Build history of the part. All positions in model axes, mm. A direction names the side the tool comes from. Give positions to 0.01 mm unless a question says otherwise; leave off trailing zeros. Order: outer loops, then holes, each group sorted by start corner. A loop starts at its lowest first (then second) coordinate and runs counter-clockwise, first axis right, second up. Notation, with made-up numbers: M -10,78 L 43,78 A35 ccw 43,110 Z; hole C -36.5,88 d8. An arc over 180 degrees is marked long. One line per item, written item: value.
from build123d import *

# Parameters (mm, degrees)
F0_W     = 42
F0_H     = 42
F1_DEPTH = 5
F3_D     = 5
F4_W     = 42
F4_H     = 5
F5_DEPTH = 5
F6_W     = 42
F6_H     = 5
F7_DEPTH = 20
F8_W     = 42
F8_H     = 5
F8_H_2   = 25
F9_DEPTH = 5
F11_D    = 5
F13_D    = 25


with BuildPart() as f1:
    # F0 (on Top) → F1 (new body)
    with BuildSketch(Plane.XY):
        Rectangle(F0_W, F0_H)
    extrude(amount=F1_DEPTH)

    # F3 (through all)
    with Locations(Plane.XY.offset(5)):
        with Locations((-15.5, 15.5), (15.5, 15.5), (15.5, -15.5), (-15.5, -15.5)):
            Hole(F3_D / 2)

    # F4 (on face) → F5 (join)
    with BuildSketch(Plane(origin=(0, 21, 0), x_dir=(-1, 0, 0), z_dir=(0, 1, 0))):
        with Locations((0, 2.5)):
            Rectangle(F4_W, F4_H)
    extrude(amount=F5_DEPTH)

    # F6 (on face) → F7 (join)
    with BuildSketch(Plane(origin=(0, 0, 0), x_dir=(1, 0, 0), z_dir=(0, 0, -1))):
        with Locations((0, -23.5)):
            Rectangle(F6_W, F6_H)
    extrude(amount=F7_DEPTH)

    # F8 (on face) → F9 (join)
    with BuildSketch(Plane(origin=(0, 0, -20), x_dir=(1, 0, 0), z_dir=(0, 0, -1))):
        with Locations((0, -23.5)):
            Rectangle(F8_W, F8_H)
        with Locations((0, -38.5)):
            Rectangle(F8_W, F8_H_2)
    extrude(amount=F9_DEPTH)

    # F11 (through all)
    with Locations(Plane(origin=(0, 0, -25), x_dir=(1, 0, 0), z_dir=(0, 0, -1))):
        with Locations((-16.56834, -31.176092), (16.56834, -31.176092), (16.56834, -45.494268), (-16.56834, -45.494268)):
            Hole(F11_D / 2)

    # F13 (through all)
    with Locations(Plane(origin=(0, 0, 0), x_dir=(1, 0, 0), z_dir=(0, 0, -1))):
        with Locations((0, 0)):
            Hole(F13_D / 2)


solid = f1.part
1) Saw through at C-C, the plane y = 0. Write the cut outline in (x, z), then the cut area to 3 significant figures.
Check values:
outline: M -21,0 L -12.5,0 L -12.5,5 L -21,5 Z; M 12.5,0 L 21,0 L 21,5 L 12.5,5 Z
area: 85.0 mm^2
2) Saw through at B-B, the plane y = -15.5. Write the cut outline in (x, z).
Check values:
outline: M -21,0 L -18,0 L -18,5 L -21,5 Z; M -13,0 L 13,0 L 13,5 L -13,5 Z; M 18,0 L 21,0 L 21,5 L 18,5 Z
3) Tool access for faces 4 (the face through (0, 26, -7)), 5 (the face through (-9, 9, 0)), 6 (the face through (-17.912, 43.386, -22.465)): list every direction of +Z, -Z, +X, -X, +Y, -Y with a clear straight run to the whole face (end or side of a thin tool).
Check values:
face 4: +Z, +X, -X, +Y
face 5: -Z, +X, -X, -Y
face 6: +Z, -Z
4) Saw through at A-A, the plane x = 0. Write the cut outline in (y, z), then the cut area to 3 significant figures.
Check values:
outline: M -21,0 L -12.5,0 L -12.5,5 L -21,5 Z; M 12.5,0 L 21,0 L 21,-25 L 51,-25 L 51,-20 L 26,-20 L 26,5 L 12.5,5 Z
area: 360 mm^2
5) Pin check, flat tips, straight feed: pin 1 (6.5 mm diameter, centred on x = 15.5, y = 15.5, fed in from -Z); pin 2 (6.5 mm diameter, centred on x = 16.57, y = 31.18, fed in from +Z); pin 3 (3 mm diameter, centred on x = 11.5, z = -18, fed in from +Y). Stop position of each tip, or through.
Check values:
pin 1: z = 0
pin 2: z = -20
pin 3: y = 26
6) Saw through at D-D, the plane x = 15.5. Write the cut outline in (y, z), then the cut area to 3 significant figures.
Check values:
outline: M -21,0 L -18,0 L -18,5 L -21,5 Z; M -13,0 L 13,0 L 13,5 L -13,5 Z; M 18,0 L 21,0 L 21,-25 L 28.92,-25 L 28.92,-20 L 26,-20 L 26,5 L 18,5 Z; M 33.44,-25 L 43.23,-25 L 43.23,-20 L 33.44,-20 Z; M 47.75,-25 L 51,-25 L 51,-20 L 47.75,-20 Z
area: 390 mm^2
7) Mould opens along X. For faces 1 (the face through (18.411, 43.805, -22.465)), 2 (the face through (0, 38, -20)), 3 (the face through (21, 23, -7)) say: released by +X, released by -X, zero draft, split by the parting line, or undercut.
Check values:
face 1: undercut
face 2: zero draft
face 3: released by +X
8) Drill centre lines: probe 1 along Y at (x, z) = (15.5, 3.2); probe 2 along Y at (x, z) = (0, 1.95); probe 3 along Z at (x, y) = (12, 47). Where is each one in solid material? Low to high. Write a range as from..to.
Check values:
probe 1: -21..-18, -13..13, 18..26
probe 2: -21..-12.5, 12.5..26
probe 3: -25..-20
